Can you work these out from the model? Positions are in its coordinate system, mm. A direction names the side the tool comes from. Give positions to 0.01 mm unless a question says otherwise; leave off trailing zeros. Loops run counter-clockwise (first coordinate to the right, second up) from the corner with the lowest first, then second, coordinate; pieces in that order, holes last. Notation, with made-up numbers: (3.25, 87.5) -> (25.25, 87.5) arc R13 ccw to (25.25, 110.5) -> close; hole circle Ø2 at (1.25, 61.5). An arc over 180 degrees is marked (long way). Return JSON: item names as keys, results as strings. Group by question number.
Q1. Suppose I cut it at D-D, the plane y = -18.5. Please give me the cut outline in (x, z).
Q2. I need wall thicknesses on line 1 along X through (y, z) = (-21.25, 0); line 2 along X through (y, z) = (33, 0); line 3 along Y through (x, z) = (-60, -71). Which ranges of each line are inside material? Lowest first, please. Write a range as [from, to].
Q3. Which directions (+Z, -Z, +X, -X, +Y, -Y) give clear straight access to the entire face, cutting with the end or side of a thin tool? Please do faces 1 (the flat face through (54, 65, 66)), 2 (the flat face through (-98, 0, -2)), 3 (the flat face through (-65, 5, 65)).
Q4. Suppose I cut it at A-A, the plane x = 0. Please give me the cut outline in (y, z).
Q5. Thinking about a two-plate mould opening in X: for faces 4 (the flat face through (-41, 0, 75)), 5 (the flat face through (36, -30, 86)), 6 (the cylindrical face through (-91.273, 2.465, -119.035)), 7 (the cylindrical face through (-90.3, -14.79, 20.05)), which applies, pulls with the +X half, pulls with the -X half, needs draft (parallel to the pull), parting line crosses it, or undercut?
Q6. Suppose I cut it at C-C, the plane y = 56. Please give me the cut outline in (x, z).
Q7. Will these pins go through, and if not, where does the flat tip stop? pin 1 (4 mm diameter, centred on x = -71.5, y = 8, fed in from -Z); pin 2 (6 mm diameter, centred on x = -103.5, y = 6.5, fed in from -Z); pin 3 (6 mm diameter, centred on x = 39, z = 88.5, fed in from +Y).
Q8. Suppose I cut it at B-B, the plane z = 0. Please give me the cut outline in (x, y), and give its area (3 significant figures).
```python
from build123d import *

# Parameters (mm, degrees)
SKETCH_2_R          = 150
EXTRUDE_1_DEPTH     = 5
SKETCH_3_R          = 90
EXTRUDE_2_DEPTH     = 60
SKETCH_4_R          = 85
CUT_EXTRUDE_1_DEPTH = 222.867077323
SKETCH_5_R          = 97.5
SKETCH_5_R_2        = 92.5
EXTRUDE_3_DEPTH     = 30


with BuildPart() as part:
    # 草图2 → 凸台-拉伸1 (new body)
    with BuildSketch(Plane(origin=(0, 0, 0), x_dir=(1, 0, 0), z_dir=(0, 1, 0))):
        with Locations(Location((0, 0, 0), (0, 0, 270))):
            Circle(SKETCH_2_R)
    extrude(amount=EXTRUDE_1_DEPTH)

    # 草图3 → 凸台-拉伸2 (add)
    with BuildSketch(Plane(origin=(0, 5, 0), x_dir=(1, 0, 0), z_dir=(0, 1, 0))):
        with Locations(Location((0, 0, 0), (0, 0, 270))):
            Circle(SKETCH_3_R)
    extrude(amount=EXTRUDE_2_DEPTH)

    # 草图4 → 切除-拉伸1 (cut, through all)
    with BuildSketch(Plane.XZ):
        with Locations(Location((0, 0, 0), (0, 0, 270))):
            Circle(SKETCH_4_R)
    extrude(amount=-CUT_EXTRUDE_1_DEPTH, mode=Mode.SUBTRACT)

    # 草图5 → 凸台-拉伸3 (add)
    with BuildSketch(Plane.XZ):
        with Locations(Location((0, 0, 0), (0, 0, 90))):
            Circle(SKETCH_5_R)
        with Locations(Location((0, 0, 0), (0, 0, 270))):
            Circle(SKETCH_5_R_2, mode=Mode.SUBTRACT)
    extrude(amount=EXTRUDE_3_DEPTH)


solid = part.part
```
Ans:
{
 "1": {"outline": "circle Ø195 at (0, 0); hole circle Ø185 at (0, 0)"},
 "2": {"line 1": "x = [-97.5, -92.5], [92.5, 97.5]", "line 2": "x = [-90, -85], [85, 90]", "line 3": "y = [-30, 5]"},
 "3": {"face 1": "+Z, -Z, +X, -X, +Y", "face 2": "-Y", "face 3": "+Y"},
 "4": {"outline": "(-30, -97.5) -> (0, -97.5) -> (0, -150) -> (5, -150) -> (5, -90) -> (65, -90) -> (65, -85) -> (0, -85) -> (0, -92.5) -> (-30, -92.5) -> close; (-30, 92.5) -> (0, 92.5) -> (0, 85) -> (65, 85) -> (65, 90) -> (5, 90) -> (5, 150) -> (0, 150) -> (0, 97.5) -> (-30, 97.5) -> close"},
 "5": {"face 4": "undercut", "face 5": "needs draft", "face 6": "parting line crosses it", "face 7": "undercut"},
 "6": {"outline": "circle Ø180 at (0, 0); hole circle Ø170 at (0, 0)"},
 "7": {"pin 1": "stops at z = -57.18", "pin 2": "stops at z = -110.99", "pin 3": "stops at y = 5"},
 "8": {"outline": "(-150, 0) -> (-97.5, 0) -> (-97.5, -30) -> (-92.5, -30) -> (-92.5, 0) -> (-85, 0) -> (-85, 65) -> (-90, 65) -> (-90, 5) -> (-150, 5) -> close; (85, 0) -> (92.5, 0) -> (92.5, -30) -> (97.5, -30) -> (97.5, 0) -> (150, 0) -> (150, 5) -> (90, 5) -> (90, 65) -> (85, 65) -> close", "area": "1,550 mm^2"}
}
